Drawing for the job (mm, zero at the part's lowest x, y, z). Round coordinates to 2 decimals unless told otherwise and drop trailing zeros. Loops run counter-clockwise (first coordinate to the right, second up) from the corner with the lowest first, then second, coordinate; pieces in that order, holes last. Notation, with made-up numbers: (43.25, 89.25) - (87.25, 89.25) arc R30 cw to (87.25, 128.25) - close; hole circle Ø3 at (8.25, 41). An arc over 180 degrees is marked (long way). Put each result on its own line as item: value.
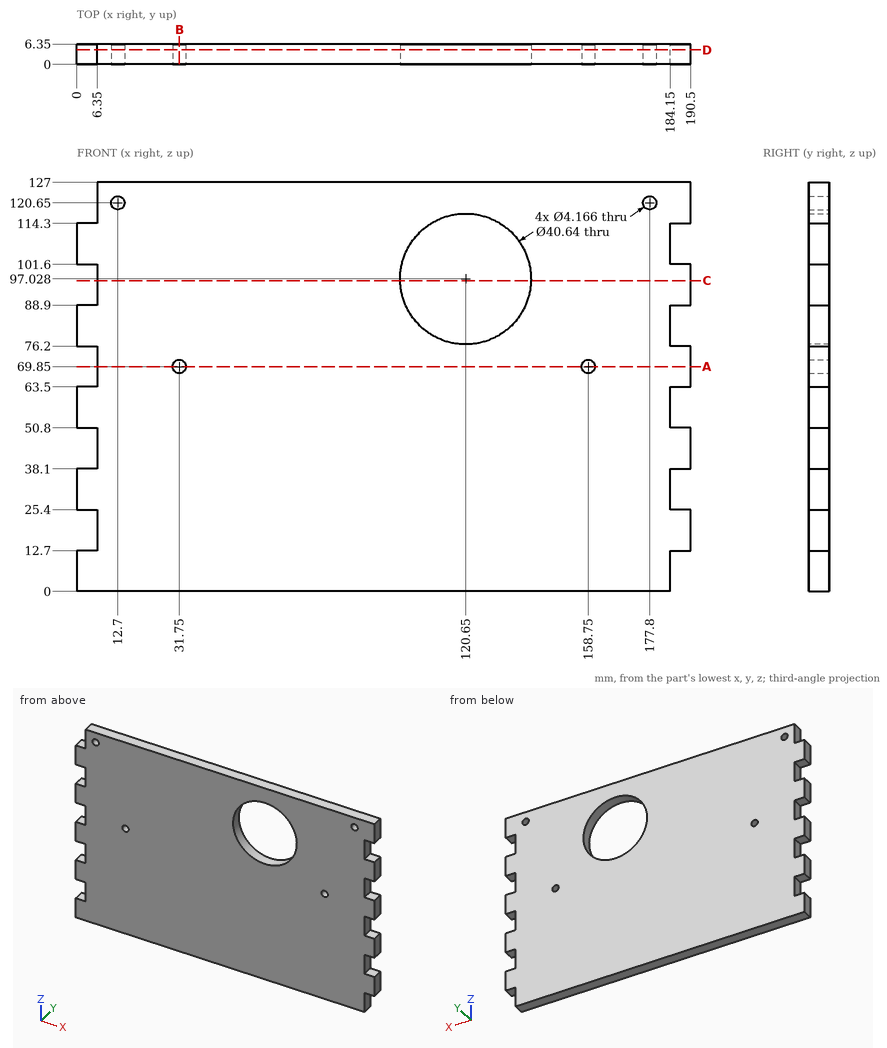
1. Band-saw the part on B-B (x = 31.75). List the corners of the cut face in (y, z), plus the area to 3 significant figures.
A:
outline: (0, 0) - (6.35, 0) - (6.35, 67.77) - (0, 67.77) - close; (0, 71.93) - (6.35, 71.93) - (6.35, 127) - (0, 127) - close
area: 780 mm²
2. Pin check, flat tips, straight feed: P1, Ø1.5, axis at y = 4.5, z = 24.5, coming from the -X side; P2, Ø3, axis at y = 2.5, z = 58, coming from the +X side; P3, Ø1.9, axis at x = 4, y = 3.5, coming from the +Z side; P4, Ø3.5, axis at x = 158.75, z = 69.85, coming from the +Y side. Stop position of each tip, or through.
A:
P1: stops at x = 6.35
P2: stops at x = 184.15
P3: stops at z = 114.3
P4: passes through
3. Band-saw the part on C-C (z = 96.5). List the corners of the cut face in (x, y).
A:
outline: (6.35, 0) - (100.34, 0) - (100.34, 6.35) - (6.35, 6.35) - close; (140.96, 0) - (190.5, 0) - (190.5, 6.35) - (140.96, 6.35) - close
4. Probe line 1 along X through (y, z) = (4, 69.85); line 2 along X through (y, z) = (3.5, 120.65); line 3 along X through (y, z) = (2.25, 9). List the from-to ranges inside material, lowest first. Write a range as [from, to].
A:
line 1: x = [6.35, 29.67], [33.83, 156.67], [160.83, 190.5]
line 2: x = [6.35, 10.62], [14.78, 175.72], [179.88, 190.5]
line 3: x = [0, 184.15]
5. Band-saw the part on D-D (y = 4.5). Give the number of separate pieces and of enclosed holes in the cut face, plus the area to 3 significant figures.
A:
separate pieces: 1
enclosed holes: 5
area: 22,000 mm²
6. Band-saw the part on A-A (z = 69.85). List the corners of the cut face in (x, y).
A:
outline: (6.35, 0) - (29.67, 0) - (29.67, 6.35) - (6.35, 6.35) - close; (33.83, 0) - (156.67, 0) - (156.67, 6.35) - (33.83, 6.35) - close; (160.83, 0) - (190.5, 0) - (190.5, 6.35) - (160.83, 6.35) - close
